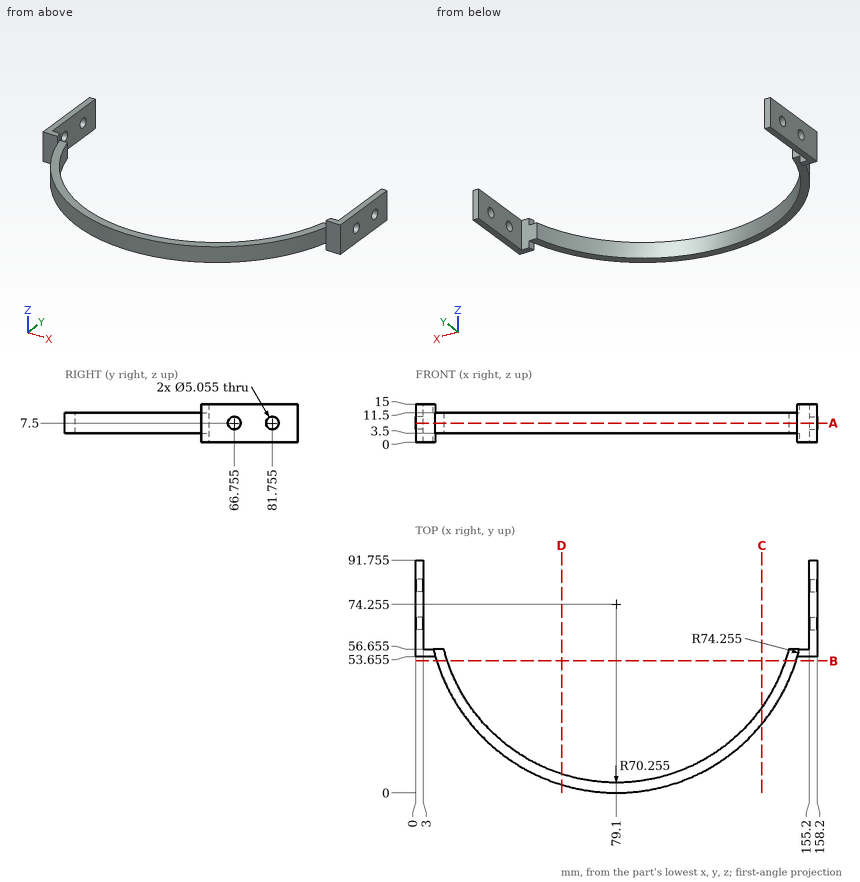
Geometry: see drawing. Coordinates: mm, zero at the bounding-box minimum. Round coordinates to 2 decimals unless told otherwise and drop trailing zeros. Loops run counter-clockwise (first coordinate to the right, second up) from the corner with the lowest first, then second, coordinate; pieces in that order, holes last. Notation, with made-up numbers: M 37.25,61 L 75.25,61 A7 ccw 75.25,74 Z; hole C 8,-34 d3. An arc over 180 degrees is marked long. Use a Markdown table: item, result. Add a question column.
1. Cut plane B-B, the plane y = 52. Output: boundary loops of the cut face in (x, z).
2. Ray query, line 1 along Y through (x, z) = (1.7, 7.5) (1 decimal); line 2 along X through (y, z) = (81, 12.75); line 3 along Y through (x, z) = (6, 4) (1 decimal). Return the intervals inside material, ascending. Write a range as [from, to].
3. Cut plane D-D, the plane x = 57.5. Output: boundary loops of the cut face in (y, z).
4. Contact query for flat-ended pins moving along their axis: pin 1 (17 mm diameter, centred on x = 74.5, y = 15.5, fed in from +Z); pin 2 (2.5 mm diameter, centred on x = 7.5, z = 6, fed in from +Y) (3 decimals); pin 3 (3 mm diameter, centred on y = 27.5, z = 7.5, fed in from +X); pin 4 (2 mm diameter, centred on y = 48, z = 11, fed in from +X). Output: stop coordinate, or through.
5. Cut plane A-A, the plane z = 7.5. Output: boundary loops of the cut face in (x, y) (1 decimal).
6. Cut plane C-C, the plane x = 136.5. Output: boundary loops of the cut face in (y, z) (1 decimal), and give its area (3 significant figures).
Solution:
| question | item | result |
|---|---|---|
| 1 | outline | M 8.26,3.5 L 12.46,3.5 L 12.46,11.5 L 8.26,11.5 Z; M 145.74,3.5 L 149.94,3.5 L 149.94,11.5 L 145.74,11.5 Z |
| 2 | line 1 | y = [53.7, 64.2], [69.3, 79.2], [84.3, 91.8] |
| 2 | line 2 | x = [0, 3], [155.2, 158.2] |
| 2 | line 3 | y = [53.7, 56.7] |
| 3 | outline | M 3.21,3.5 L 7.4,3.5 L 7.4,11.5 L 3.21,11.5 Z |
| 4 | pin 1 | passes through |
| 4 | pin 2 | stops at y = 56.655 |
| 4 | pin 3 | stops at x = 137.97 |
| 4 | pin 4 | stops at x = 148.93 |
| 5 | outline | M 0,53.7 L 7.8,53.7 A74.3 ccw 150.4,53.7 L 158.2,53.7 L 158.2,64.2 L 155.2,64.2 L 155.2,56.7 L 147.1,56.7 A70.3 cw 11.1,56.7 L 3,56.7 L 3,64.2 L 0,64.2 Z; M 0,69.3 L 3,69.3 L 3,79.2 L 0,79.2 Z; M 0,84.3 L 3,84.3 L 3,91.8 L 0,91.8 Z; M 155.2,69.3 L 158.2,69.3 L 158.2,79.2 L 155.2,79.2 Z; M 155.2,84.3 L 158.2,84.3 L 158.2,91.8 L 155.2,91.8 Z |
| 6 | outline | M 27.1,3.5 L 33.7,3.5 L 33.7,11.5 L 27.1,11.5 Z |
| 6 | area | 52.8 mm2 |
